Work out the finished part from the listing and answer in its coordinate system (mm). Face numbers are marked on the shaded views. Coordinates: 2 decimals unless noted, no trailing zeros. Answer as a JSON object with one key per item and string values. Group by question number.
1) Each of these flat-tipped pins is pushed along its axis until it touches: P1, Ø5, axis at x = 110, y = -68, coming from the -Z side; P2, Ø4, axis at x = 97.5, z = -23, coming from the +Y side; P3, Ø1, axis at y = -55, z = -8, coming from the +X side; P4, Ø12, axis at x = 144.5, y = -15, coming from the +Z side. Where does it stop, or does it pass through?
2) The mould has two halves that part along X. Classify the marked faces 1 and 2: released by +X, released by -X, zero draft, split by the parting line, or undercut.
3) Find the intervals of material crossed by line 1 along Z through (x, y) = (90.5, -55.5); line 2 along X through (y, z) = (-60, -15); line 3 along X through (y, z) = (-80.5, -16.5), in increasing order.
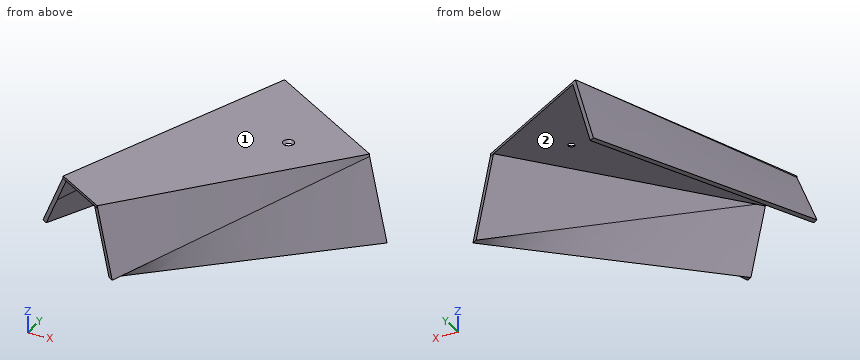
from build123d import *

# Parameters (mm, degrees)
BOSS_EXTRUDE1_DEPTH                               = 1
CSK_FOR_1_FLAT_HEAD_SOCKET_CAP_SCREW1_D           = 2.0574
CSK_FOR_1_FLAT_HEAD_SOCKET_CAP_SCREW1_CSINK_D     = 4.2672
CSK_FOR_1_FLAT_HEAD_SOCKET_CAP_SCREW1_CSINK_ANGLE = 82


with BuildPart() as part:
    # Sketch1 → Boss-Extrude1 (new body)
    with BuildSketch(Plane.XY):
        Polygon((99.80287108, 7.560475543), (62.236469572, -86.777626616), (82.236469572, -99.136126436), (149.80287108, -23.335774006), align=None)
    extrude(amount=BOSS_EXTRUDE1_DEPTH)

    # Loft3: read off the stored shape, not the designer's step
    # Loft3: loft between two sections, ruled curve by curve
    loft3_from = [
        Edge.make_bspline([(158.179985747, -28.512202511, -29), (158.486913307, -28.701860721, -29), (158.793840868, -28.891518931, -29), (159.407695988, -29.270835351, -29), (159.714623549, -29.460493561, -29), (160.021551109, -29.650151771, -29)], [0, 0, 0, 0, 0.5, 0.5, 1, 1, 1, 1], 3),
        Edge.make_bspline([(147.608937441, -21.980087582, 1), (149.370778826, -23.068773403, -4), (151.13262021, -24.157459225, -9), (154.656302978, -26.334830868, -19), (156.418144363, -27.423516689, -24), (158.179985747, -28.512202511, -29)], [0, 0, 0, 0, 0.5, 0.5, 1, 1, 1, 1], 3),
        Edge.make_bspline([(160.021551109, -29.650151771, -29), (158.318437771, -28.597755477, -24.166666667), (156.615324433, -27.545359183, -19.333333333), (153.209097757, -25.440566594, -9.666666667), (151.505984418, -24.3881703, -4.833333333), (149.80287108, -23.335774006, 0)], [0, 0, 0, 0, 0.5, 0.5, 1, 1, 1, 1], 3),
        Edge.make_bspline([(149.80287108, -23.335774006, 0), (149.80287108, -23.335774006, 0.166666667), (149.80287108, -23.335774006, 0.333333333), (149.80287108, -23.335774006, 0.666666667), (149.80287108, -23.335774006, 0.833333333), (149.80287108, -23.335774006, 1)], [0, 0, 0, 0, 0.5, 0.5, 1, 1, 1, 1], 3),
        Edge.make_line((149.80287108, -23.335774006, 1), (147.608937441, -21.980087582, 1)),
    ]
    loft3_to = [
        Edge.make_bspline([(80.395510173, -97.998551616, 0.998280313), (81.863610332, -98.905727394, -3.168099739), (83.331710492, -99.812903172, -7.334479791), (86.267910812, -101.627254727, -15.667239896), (87.736010971, -102.534430505, -19.833619948), (89.204111131, -103.441606283, -24)], [0, 0, 0, 0, 0.5, 0.5, 1, 1, 1, 1], 3),
        Edge.make_bspline([(80.395510173, -97.998551616, 1), (80.395510173, -97.998551616, 0.99971966), (80.395510173, -97.998551616, 0.999436182), (80.395510173, -97.998551616, 0.998862953), (80.395510173, -97.998551616, 0.998573202), (80.395510173, -97.998551616, 0.998280313)], [0, 0, 0, 0, 0.5, 0.5, 1, 1, 1, 1], 3),
        Edge.make_bspline([(89.204111131, -103.441606283, -24), (89.511038691, -103.631264493, -24), (89.817966252, -103.820922703, -24), (90.431821372, -104.200239123, -24), (90.738748933, -104.389897333, -24), (91.045676493, -104.579555543, -24)], [0, 0, 0, 0, 0.5, 0.5, 1, 1, 1, 1], 3),
        Edge.make_bspline([(91.045676493, -104.579555543, -24), (89.57747534, -103.672317359, -19.833333333), (88.109274186, -102.765079174, -15.666666667), (85.172871879, -100.950602805, -7.333333333), (83.704670725, -100.04336462, -3.166666667), (82.236469572, -99.136126436, 1)], [0, 0, 0, 0, 0.5, 0.5, 1, 1, 1, 1], 3),
        Edge.make_line((82.236469572, -99.136126436, 1), (80.395510173, -97.998551616, 1)),
    ]
    loft3 = Solid(Shell([*[Face.make_surface_from_curves(loft3_from[k], loft3_to[k]) for k in range(5)], Face(Wire(loft3_from)), Face(Wire(loft3_to))]))
    add(loft3)

    # Sketch12 → Loft4 section 0
    with BuildSketch(Plane(origin=(30.958675209, 50.101024656, 0), x_dir=(0.8506922729426725, -0.5256640150853298, 0), z_dir=(0.5256640150853298, 0.8506922729426725, 0))):
        with BuildLine():
            Line((82.677832154, -1), (82.677832154, 0))
            Line((82.677832154, 0), (70.665638845, 29))
            Line((70.665638845, 29), (68.500854444, 29))
            Line((68.500854444, 29), (80.927261316, -1))
            Line((80.927261316, -1), (82.677832154, -1))
        make_face()
    # Sketch13 → Loft4 section 1
    with BuildSketch(Plane(origin=(-21.6077263, -34.968202638, 0), x_dir=(-0.8506922729426724, 0.52566401508533, 0), z_dir=(-0.52566401508533, -0.8506922729426724, 0))):
        with BuildLine():
            Line((-98.864477851, -1), (-84.60323453, 24))
            Line((-84.60323453, 24), (-86.905766091, 24))
            Line((-86.905766091, 24), (-94.44679393, 10.780556805))
            Line((-94.44679393, 10.780556805), (-101.167009412, -1))
            Line((-101.167009412, -1), (-98.864477851, -1))
        make_face()
    loft()

    # CSK for #1 Flat Head Socket Cap Screw1 (through all)
    with Locations(Plane.XY.offset(1)):
        with Locations((121.150579346, -29.757979407)):
            CounterSinkHole(CSK_FOR_1_FLAT_HEAD_SOCKET_CAP_SCREW1_D / 2, CSK_FOR_1_FLAT_HEAD_SOCKET_CAP_SCREW1_CSINK_D / 2, counter_sink_angle=CSK_FOR_1_FLAT_HEAD_SOCKET_CAP_SCREW1_CSINK_ANGLE)


solid = part.part
Report:
{
 "1": {"P1": "stops at z = -10.78", "P2": "stops at y = -91.3", "P3": "stops at x = 126.72", "P4": "stops at z = 1"},
 "2": {"face 1": "zero draft", "face 2": "undercut"},
 "3": {"line 1": "z = 0 to 1", "line 2": "x = 64.19 to 66.4, 122.71 to 125.22", "line 3": "x = 54.52 to 56.96, 105.81 to 108.25"}
}
